The drawing under review shows one solid part. Ordinate dimensions are in mm from its lowest x, y, z. A direction names the side the tool comes from. Round coordinates to 2 decimals unless told otherwise and drop trailing zeros. One line per item, written item: value. Start each with the question number.
1) For P1, Ø2, axis at x = 4, y = 4, coming from the -Z side; P2, Ø3, axis at y = 12.5, z = 5.5, coming from the -X side, all flat-tipped, find the tip position at first contact; note any pin that passes through.
2) Tool access review of the marked faces 1 and 2: name each direction out of +Z, -Z, +X, -X, +Y, -Y from which nothing blocks a thin tool from reaching the whole face with its end or side.
3) Take a section at A-A, the plane x = 4.5. State how many separate pieces and enclosed holes the cut face has.
4) Wall thickness on probe 1 along X at (y, z) = (52.5, 4); probe 2 along Y at (x, z) = (2.25, 5.75) (1 decimal); probe 3 along Z at (x, y) = (5.75, 41): over which ranges is each line inside the solid? List them lowest first.
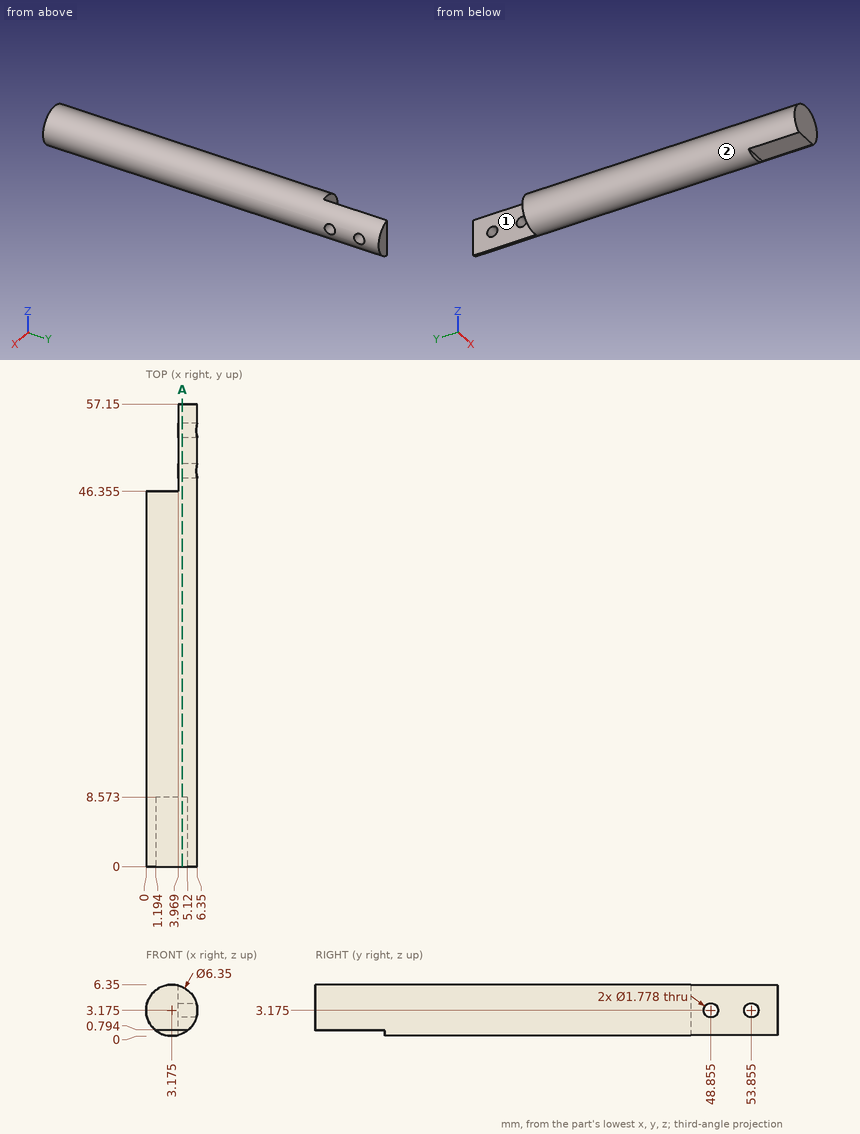
Checked values:
1. P1: stops at z = 0.79
1. P2: stops at x = 0.11
2. face 1: +Z, -Z, -X, +Y
2. face 2: +Y, -Y
3. separate pieces: 1
3. enclosed holes: 2
4. probe 1: x = 3.97 to 6.24
4. probe 2: y = 0 to 46.4
4. probe 3: z = 1.32 to 5.03
